from build123d import *

# Parameters (mm, degrees)
BOSS_EXTRUDE1_DEPTH = 10
BOSS_EXTRUDE2_DEPTH = 2
SKETCH4_R           = 4.285
SKETCH4_R_2         = 2.78
SKETCH4_R_3         = 3.175
CUT_EXTRUDE1_DEPTH  = 50.799598392
SKETCH5_R           = 1.5
CUT_EXTRUDE2_DEPTH  = 65.124878168


with BuildPart() as part:
    # Sketch2 → Boss-Extrude1 (new, symmetric)
    with BuildSketch(Plane(origin=(0, 0, 0), x_dir=(0, 0, -1), z_dir=(1, 0, 0))):
        Polygon((-44, 0), (0, 0), (0, -20), (5, -20), (5, 15), (-44, 15), align=None)
    extrude(amount=BOSS_EXTRUDE1_DEPTH, both=True)

    # Sketch3 → Boss-Extrude2 (add)
    with BuildSketch(Plane(origin=(10, 0, 0), x_dir=(0, 0, -1), z_dir=(1, 0, 0))):
        Polygon((-44, 15), (-44, -4), (-15, -4), (-15, -20), (5, -20), (5, 15), align=None)
    boss_extrude2 = extrude(amount=BOSS_EXTRUDE2_DEPTH)

    # Mirror1: Boss-Extrude2 across plane
    add(boss_extrude2.mirror(Plane(origin=(0, 0, 0), x_dir=(0, 0, 1), z_dir=(1, 0, 0))))

    # Sketch4 → Cut-Extrude1 (cut, through all)
    with BuildSketch(Plane.XZ):
        with Locations(Location((0, 34, 0), (0, 0, 270))):
            Circle(SKETCH4_R)
        with Locations(Location((0, 19, 0), (0, 0, 270))):
            Circle(SKETCH4_R_2)
        with Locations(Location((0, 7, 0), (0, 0, 270))):
            Circle(SKETCH4_R_3)
    extrude(amount=-CUT_EXTRUDE1_DEPTH, mode=Mode.SUBTRACT)

    # Sketch5 → Cut-Extrude2 (cut, through all)
    with BuildSketch(Plane(origin=(12, 0, -12), x_dir=(0, 0, 1), z_dir=(-1, 0, 0))):
        with Locations(Location((19, -10, 0), (0, 0, 180))):
            Circle(SKETCH5_R)
    extrude(amount=CUT_EXTRUDE2_DEPTH, mode=Mode.SUBTRACT)


solid = part.part
For this review, take the finished solid that the model builds, in its own axes (mm). A direction names the side the tool comes from. Give positions to 0.01 mm unless a question says otherwise; leave off trailing zeros. Order: outer loops, then holes, each group sorted by start corner. A loop starts at its lowest first (then second) coordinate and runs counter-clockwise, first axis right, second up. Notation, with made-up numbers: M 25.5,56.5 L 52.5,56.5 A25 cw 52.5,94.5 Z; hole C 52.25,74.25 d10. An arc over 180 degrees is marked long. Answer in a Markdown table with one row per item. Add a question column.
(1) Wall thickness on probe 1 along X at (y, z) = (4, 34) (3 decimals); probe 2 along X at (y, z) = (-0.5, 17); probe 3 along Y at (x, z) = (-11.05, 7): over which ranges is each line inside the solid? List them lowest first. Write a range as [from, to].
(2) Consider section B-B on z = 7. State the section outline as (x, y) points (3 decimals), and give its area (3 significant figures).
(3) Consider section C-C on x = 0. State the section outline as (y, z) points (3 decimals), and give its area (3 significant figures).
(4) For faces 4 (the face through (11, -12, 15)), 5 (the face through (0, -3, -5)), 6 (the face through (10, -8, 13)), list the 3-axis set-ups (+Z, -Z, +X, -X, +Y, -Y) from which the entire face can be reached by the end or side of a thin tool; tool diameter is ignored.
(5) Consider section A-A on z = 34. State the section outline as (x, y) points (3 decimals).
(6) Mouldability with a two-part tool opening along Z and no side actions: class faces 1 (the face through (-11, -9.1, 8.2)), 2 (the face through (-11, -12, 15)), 3 (the face through (-11, -4, 30)) as +Z half, -Z half, draft (parallel to the pull), parting line (faces both ways), or undercut.
(7) Consider section D-D on y = -5. State the section outline as (x, z) points, and give its area (3 significant figures).
(8) For pin 1 (1.6 mm diameter, centred on x = -10.5, y = -16, fed in from +Z); pin 2 (5 mm diameter, centred on x = 0, z = 34, fed in from -Y) (3 decimals); pin 3 (6 mm diameter, centred on x = -0.5, y = -14, fed in from +Z); pin 4 (6 mm diameter, centred on x = 2.5, z = 17, fed in from -Y), all flat-tipped, find the tip position at first contact; note any pin that passes through.
Evaluation:
| question | item | result |
|---|---|---|
| 1 | probe 1 | x = [-12, -4.285], [4.285, 12] |
| 1 | probe 2 | x = [-12, -10], [10, 12] |
| 1 | probe 3 | y = [-20, -11.5], [-8.5, 15] |
| 2 | outline | M -12,-20 L -10,-20 L -10,-11.5 L -12,-11.5 Z; M -12,-8.5 L -10,-8.5 L -10,0 L -3.175,0 L -3.175,15 L -12,15 Z; M 3.175,0 L 10,0 L 10,-8.5 L 12,-8.5 L 12,15 L 3.175,15 Z; M 10,-20 L 12,-20 L 12,-11.5 L 10,-11.5 Z |
| 2 | area | 333 mm^2 |
| 3 | outline | M -20,-5 L 15,-5 L 15,3.825 L 0,3.825 L 0,0 L -20,0 Z; M 0,10.175 L 15,10.175 L 15,16.22 L 0,16.22 Z; M 0,21.78 L 15,21.78 L 15,29.715 L 0,29.715 Z; M 0,38.285 L 15,38.285 L 15,44 L 0,44 Z |
| 3 | area | 528 mm^2 |
| 4 | face 4 | +Z, +X, -X, -Y |
| 4 | face 5 | -Z, +X, -X, +Y, -Y |
| 4 | face 6 | +Z, -Y |
| 5 | outline | M -12,-4 L -10,-4 L -10,0 L -4.285,0 L -4.285,15 L -12,15 Z; M 4.285,0 L 10,0 L 10,-4 L 12,-4 L 12,15 L 4.285,15 Z |
| 6 | face 1 | undercut |
| 6 | face 2 | +Z half |
| 6 | face 3 | draft |
| 7 | outline | M -12,-5 L 12,-5 L 12,15 L 10,15 L 10,0 L -10,0 L -10,15 L -12,15 Z |
| 7 | area | 180 mm^2 |
| 8 | pin 1 | stops at z = 15 |
| 8 | pin 2 | passes through |
| 8 | pin 3 | stops at z = 0 |
| 8 | pin 4 | stops at y = 0 |
